Autodesk Inventor part; units mm, degrees
ref_plane "YZ Plane" through (0, 0, 0) normal (1, 0, 0) x (0, 1, 0)
ref_plane "XZ Plane" through (0, 0, 0) normal (0, 1, 0) x (-1, 0, 0)
ref_plane "XY Plane" through (0, 0, 0) normal (0, 0, 1) x (1, 0, 0)
sketch "Szkic1" plane through (0, 0, 0) normal (0, 0, 1) x (1, 0, 0)
  line L0 (0, 0) -> (-8, 0)
  line L1 (-8, 0) -> (-8, 8)
  line L2 (-8, 8) -> (0, 8)
  line L3 (0, 8) -> (0, 0)
  dimension "d0" = 8
  dimension "d1" = 8
extrude "Wyciągnięcie proste1" add sketch "Szkic1" along normal blind 5
sketch "Szkic2" plane through (0, 0, 0) normal (0, 0, -1) x (-1, 0, 0)
  line L0 (0, 8) -> (8, 8)
  line L1 (4, 8) -> (4, 0)
  line L2 (8, 0) -> (0, 0)
  line L3 (0, 0) -> (0, 8)
  line L4 (0, 4) -> (8, 4)
  line L5 (8, 8) -> (8, 0)
  point P0 (4, 4)
hole "Otwór1" at (-4, 4, 0) direction (0, 0, 1) diameter 2.459 end through all
properties part number "zatyczka na szyne" material "Stal nierdzewna 440C"
Can you work these out from the model? Positions are in its coordinate system, mm. Coordinates: 2 decimals unless noted, no trailing zeros. Loops run counter-clockwise (first coordinate to the right, second up) from the corner with the lowest first, then second, coordinate; pieces in that order, holes last. Notation, with made-up numbers: M 63,47.5 L 104,47.5 A28 cw 104,67.5 Z; hole C 61,63.25 d7. An arc over 180 degrees is marked long. Put each result on its own line as item: value. Start each with the question number.
(1) We'd pull the mould along Y, two halves only. Please class faces 1 (the face through (-4.05, 2.77, 2.54)), 2 (the face through (-4, 0, 2)), 3 (the face through (-4, 8, 2)): +Y half, -Y half, draft (parallel to the pull), parting line (faces both ways), or undercut.
(2) I need wall thicknesses on probe 1 along Y at (x, z) = (-4, 3.05); probe 2 along X at (y, z) = (4, 2.2); probe 3 along Y at (x, z) = (-4.5, 1). Which ranges of each line are inside material? Lowest first, please.
(3) Will this pin go through, and if not, where does the flat tip stop? pin 1 Ø2 at (x, y) = (-6, 6.5) entering from -Z.
(4) Imagine slicing it at B-B on y = 4. List the corners of the cut face in (x, z) for me, and give its area (3 significant figures).
(5) Imagine slicing it at C-C on z = 4.7. List the corners of the cut face in (x, y) for me.
(6) Imagine slicing it at A-A on x = -4. List the corners of the cut face in (y, z) for me.
Worked answers:
1. face 1: undercut
1. face 2: -Y half
1. face 3: +Y half
2. probe 1: y = 0 to 2.77, 5.23 to 8
2. probe 2: x = -8 to -5.23, -2.77 to 0
2. probe 3: y = 0 to 2.88, 5.12 to 8
3. pin 1: stops at z = 0
4. outline: M -8,0 L -5.23,0 L -5.23,5 L -8,5 Z; M -2.77,0 L 0,0 L 0,5 L -2.77,5 Z
4. area: 27.7 mm2
5. outline: M -8,0 L 0,0 L 0,8 L -8,8 Z; hole C -4,4 d2.46
6. outline: M 0,0 L 2.77,0 L 2.77,5 L 0,5 Z; M 5.23,0 L 8,0 L 8,5 L 5.23,5 Z
